```python
from build123d import *

# Parameters (mm, degrees)
SKETCH_W        = 50
SKETCH_H        = 100
PAD_DEPTH       = 40
SKETCH001_W     = 40
SKETCH001_H     = 90
POCKET_DEPTH    = 35
SKETCH002_W     = 40
SKETCH002_H     = 25
POCKET001_DEPTH = 5.001
SKETCH003_W     = 40
SKETCH003_H     = 25
POCKET002_DEPTH = 5.001
SKETCH004_R     = 5
POCKET003_DEPTH = 100.001


with BuildPart() as part:
    # Sketch → Pad (new body)
    with BuildSketch(Plane.XY):
        with Locations((25, 50)):
            Rectangle(SKETCH_W, SKETCH_H)
    extrude(amount=PAD_DEPTH)

    # Sketch001 (on Face6 of Pad) → Pocket (cut)
    with BuildSketch(Plane.XY.offset(40)):
        with Locations((25, 50)):
            Rectangle(SKETCH001_W, SKETCH001_H)
    extrude(amount=-POCKET_DEPTH, mode=Mode.SUBTRACT)

    # Sketch002 (on Face11 of Pocket) → Pocket001 (cut, through all)
    with BuildSketch(Plane.XY.offset(5)):
        with Locations((25, 82.5)):
            Rectangle(SKETCH002_W, SKETCH002_H)
    extrude(amount=-POCKET001_DEPTH, mode=Mode.SUBTRACT)

    # Sketch003 (on Face9 of Pocket001) → Pocket002 (cut, through all)
    with BuildSketch(Plane.XY.offset(5)):
        with Locations((25, 17.5)):
            Rectangle(SKETCH003_W, SKETCH003_H)
    extrude(amount=-POCKET002_DEPTH, mode=Mode.SUBTRACT)

    # Sketch004 (on Face1 of Pocket002) → Pocket003 (cut, through all)
    with BuildSketch(Plane.XZ):
        with Locations((15, 27.5)):
            Circle(SKETCH004_R)
        with Locations((35, 27.5)):
            Circle(SKETCH004_R)
    extrude(amount=-POCKET003_DEPTH, mode=Mode.SUBTRACT)


solid = part.part
```
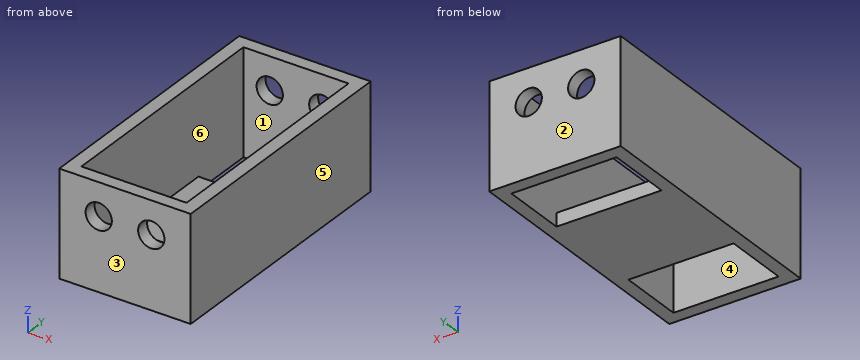
Here's how the part is built. I have some questions about the finished solid (model axes, mm). Face numbers are marked on the shaded views. A direction names the side the tool comes from. Give positions to 0.01 mm unless a question says otherwise; leave off trailing zeros. Loops run counter-clockwise (first coordinate to the right, second up) from the corner with the lowest first, then second, coordinate; pieces in that order, holes last. Notation, with made-up numbers: (78, -34.5) -> (131, -34.5) arc R15 cw to (131, -8.5) -> close; hole circle Ø3 at (-13, 19). An arc over 180 degrees is marked (long way). Use one line per item in the form item = value. Start each with the question number.
1) Imagine slicing it at A-A (y = 91.5). Please give me the cut outline in (x, z).
2) Thinking about a two-plate mould opening in Y: for the marked faces 1, 2, 3 and 4, which applies, +Y half, -Y half, draft (parallel to the pull), parting line (faces both ways), or undercut?
3) For P1, Ø12, axis at x = 30, y = 35, coming from the -Z side; P2, Ø20, axis at x = 33.5, y = 41.5, coming from the +Z side, each with a flat end and sliding along its axis, tell me the tip position at first contact or that it passes through.
4) Imagine slicing it at B-B (x = 15). Please give me the cut outline in (y, z).
5) Please list where these lines run through material, in increasing order: line 1 along Y through (x, z) = (19, 2); line 2 along X through (y, z) = (66, 16); line 3 along Y through (x, z) = (11.5, 10).
6) Which directions (+Z, -Z, +X, -X, +Y, -Y) give clear straight access to the entire face, cutting with the end or side of a thin tool? Please do the marked faces 5 and 6.
7) Imagine slicing it at D-D (y = 53.5). Please give me the cut outline in (x, z).
8) Imagine slicing it at C-C (z = 27.5). Please give me the cut outline in (x, y), then the cut area to 3 significant figures.
Check values:
q1.outline = (0, 0) -> (5, 0) -> (5, 40) -> (0, 40) -> close; (45, 0) -> (50, 0) -> (50, 40) -> (45, 40) -> close
q2.face_1 = undercut
q2.face_2 = +Y half
q2.face_3 = -Y half
q2.face_4 = undercut
q3.P1 = 0
q3.P2 = 5
q4.outline = (0, 0) -> (5, 0) -> (5, 22.5) -> (0, 22.5) -> close; (0, 32.5) -> (5, 32.5) -> (5, 40) -> (0, 40) -> close; (30, 0) -> (70, 0) -> (70, 5) -> (30, 5) -> close; (95, 0) -> (100, 0) -> (100, 22.5) -> (95, 22.5) -> close; (95, 32.5) -> (100, 32.5) -> (100, 40) -> (95, 40) -> close
q5.line_1 = 0 to 5, 30 to 70, 95 to 100
q5.line_2 = 0 to 5, 45 to 50
q5.line_3 = 0 to 5, 95 to 100
q6.face_5 = +Z, -Z, +X, +Y, -Y
q6.face_6 = +Z
q7.outline = (0, 0) -> (50, 0) -> (50, 40) -> (45, 40) -> (45, 5) -> (5, 5) -> (5, 40) -> (0, 40) -> close
q8.outline = (0, 0) -> (10, 0) -> (10, 5) -> (5, 5) -> (5, 95) -> (10, 95) -> (10, 100) -> (0, 100) -> close; (20, 0) -> (30, 0) -> (30, 5) -> (20, 5) -> close; (20, 95) -> (30, 95) -> (30, 100) -> (20, 100) -> close; (40, 0) -> (50, 0) -> (50, 100) -> (40, 100) -> (40, 95) -> (45, 95) -> (45, 5) -> (40, 5) -> close
q8.area = 1,200 mm^2
